Verification items for the finished model (mm, model axes). Face numbers are marked on the shaded views. A direction names the side the tool comes from. Give positions to 0.01 mm unless a question says otherwise; leave off trailing zeros. Write each loop counter-clockwise with the first axis right and the second up, starting at its lowest first coordinate (ties: lowest second). Pieces come first, ordered by that corner, then holes. Notation, with made-up numbers: (85.5, 87.25) - (99.5, 87.25) arc R28 cw to (99.5, 105.25) - close; hole circle Ø8 at (83.25, 79.25). An arc over 180 degrees is marked (long way). Answer as a JSON object with one key per item and string values. Group by question number.
Item 1: Sectioned sample at D-D, the plane x = -18. Record the boundary of the cut face in (y, z), and give its area (3 significant figures).
Item 2: Sectioned sample at B-B, the plane y = -31. Count the separate pieces of the cut face and the enclosed holes in it, and give its area (3 significant figures).
Item 3: Go/stop test with flat-tipped pins: pin 1 (3 mm diameter, centred on x = 11, z = -0.5, fed in from +Y); pin 2 (1.3 mm diameter, centred on y = -13.5, z = 0, fed in from -X); pin 3 (10 mm diameter, centred on x = -13.5, y = -12, fed in from -Z); pin 4 (2 mm diameter, centred on x = 6.5, y = -23, fed in from -Z). Record where each tip stops, or that it passes through.
Item 4: Tool access check on the marked faces 1 and 2. Record the directions out of +Z, -Z, +X, -X, +Y, -Y that give a thin tool (end or side, any length) a straight path to the whole face; none if there is none.
Item 5: Sectioned sample at C-C, the plane x = -9.5. Record the boundary of the cut face in (y, z).
Item 6: Sectioned sample at A-A, the plane z = -3.1. Record the boundary of the cut face in (x, y) (3 decimals), and give its area (3 significant figures).
Item 7: Scan lines: line 1 along Y through (x, z) = (9.5, 0.7); line 2 along Y through (x, z) = (22.5, -2.2); line 3 along Y through (x, z) = (-22, -3.05). Record each from-to range of solid material in increasing order. Write a range as [from, to].
```python
from build123d import *

# Parameters (mm, degrees)
F1_DEPTH    = 44.45
F2_R        = 5.07999
F3_R        = 1.397
F4_DEPTH    = 25.4
F5_W        = 15.24
F5_H        = 11.5777312835
F6_DEPTH    = 25.4
F7_R        = 2.54
F8_T1_DEPTH = 50.9820747894


# Not quite as in the source:
# - a fillet or chamfer that OpenCascade refuses, or shapes differently, is made with other operations: its cross-section is extruded or revolved along the edge and cut away or added
# - a fillet or chamfer is up to 0.001 mm smaller than in the source, because OpenCascade refuses the exact size


with BuildPart() as f1:
    # F0 (on Front) → F1 (new body)
    with BuildSketch(Plane.XZ):
        Polygon((0, 1.27), (-25.4, 1.27), (-25.4, -1.27), (-25.4, -3.81), (-19.05, -3.81), (-19.05, -1.27), (19.05, -1.27), (19.05, -3.81), (25.4, -3.81), (25.4, -1.27), (25.4, 1.27), align=None)
    extrude(amount=F1_DEPTH)

    # F2 (radius 5.08 in the source; OpenCascade refuses exactly that, so slightly less here)
    f2_edges = [f1.edges().sort_by_distance(p)[0] for p in [
        (-25.4, -22.225, 1.27),
        (25.4, -22.225, 1.27),
    ]]
    fillet(f2_edges, radius=F2_R)

    # F3 (on face) → F4 (cut)
    with BuildSketch(Plane(origin=(0, 0, -3.81), x_dir=(1, 0, 0), z_dir=(0, 0, -1))):
        with BuildLine():
            ThreePointArc((-22.225, 23.622), (-23.2128281733, 21.2371718267), (-20.828, 22.225))
            Line((-20.828, 22.225), (-22.225, 22.225))
            Line((-22.225, 22.225), (-22.225, 23.622))
        make_face()
        with BuildLine():
            Line((-22.225, 22.225), (-20.828, 22.225))
            ThreePointArc((-20.828, 22.225), (-21.2371718267, 23.2128281733), (-22.225, 23.622))
            Line((-22.225, 23.622), (-22.225, 22.225))
        make_face()
        with BuildLine():
            ThreePointArc((-22.225, 42.672), (-23.622, 41.275), (-22.225, 39.878))
            Line((-22.225, 39.878), (-22.225, 41.275))
            Line((-22.225, 41.275), (-22.225, 42.672))
        make_face()
        with BuildLine():
            Line((-22.225, 41.275), (-22.225, 39.878))
            ThreePointArc((-22.225, 39.878), (-21.2371718267, 40.2871718267), (-20.828, 41.275))
            ThreePointArc((-20.828, 41.275), (-21.2371718267, 42.2628281733), (-22.225, 42.672))
            Line((-22.225, 42.672), (-22.225, 41.275))
        make_face()
        with Locations((-22.225, 3.175)):
            Circle(F3_R)
        with Locations((22.225, 41.275)):
            Circle(F3_R)
        with Locations((22.225, 3.175)):
            Circle(F3_R)
        with Locations((22.225, 22.225)):
            Circle(F3_R)
    extrude(amount=-F4_DEPTH, mode=Mode.SUBTRACT)

    # F5 (on face) → F6 (cut)
    with BuildSketch(Plane.XY.offset(1.27)):
        with Locations((11.43, -12.1388656418)):
            Rectangle(F5_W, F5_H)
        with Locations((-11.43, -12.1388656418)):
            Rectangle(F5_W, F5_H)
        with Locations((11.43, -32.3111343582)):
            Rectangle(F5_W, F5_H)
        with Locations((-11.43, -32.3111343582)):
            Rectangle(F5_W, F5_H)
    extrude(amount=-F6_DEPTH, mode=Mode.SUBTRACT)

    # F7
    f7_edges = [f1.edges().sort_by_distance(p)[0] for p in [
        (-19.05, -6.35, 0),
        (-3.81, -17.927731, 0),
        (-3.81, -6.35, 0),
        (-19.05, -17.927731, 0),
        (-19.05, -38.1, 0),
        (3.81, -38.1, 0),
        (3.81, -17.927731, 0),
        (3.81, -6.35, 0),
        (-19.05, -26.522269, 0),
        (3.81, -26.522269, 0),
        (19.05, -26.522269, 0),
        (-3.81, -26.522269, 0),
        (19.05, -6.35, 0),
        (19.05, -17.927731, 0),
        (19.05, -38.1, 0),
        (-3.81, -38.1, 0),
    ]]
    fillet(f7_edges, radius=F7_R)

    # F8: chamfer of 1.27 on 14 edges, made by hand

    # F8_s2 → F8_t1 (cut)
    with BuildSketch(Plane.XZ.offset(-3.2660373947)):
        Polygon((19.05, -2.54), (20.32, -3.81), (19.05, -3.81), align=None)
        Polygon((-19.05, -2.54), (-20.32, -3.81), (-19.05, -3.81), align=None)
    extrude(amount=F8_T1_DEPTH, mode=Mode.SUBTRACT)


solid = f1.part
```
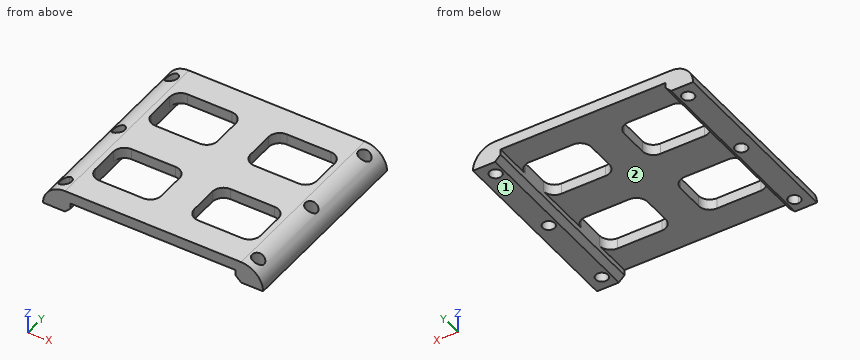
Geometry check:
{
 "1": {"outline": "(-44.45, -1.27) - (-37.62, -1.27) - (-37.62, 1.27) - (-44.45, 1.27) - close; (-27.01, -1.27) - (-17.44, -1.27) - (-17.44, 1.27) - (-27.01, 1.27) - close; (-6.83, -1.27) - (0, -1.27) - (0, 1.27) - (-6.83, 1.27) - close", "area": "59.0 mm^2"},
 "2": {"separate pieces": "3", "enclosed holes": "0", "area": "71.2 mm^2"},
 "3": {"pin 1": "y = 0", "pin 2": "x = -24.3", "pin 3": "through", "pin 4": "z = -1.27"},
 "4": {"face 1": "-Z, +X, -X, +Y, -Y", "face 2": "-Z, +Y, -Y"},
 "5": {"outline": "(-44.45, -1.27) - (-38.1, -1.27) - (-38.1, 1.27) - (-44.45, 1.27) - close; (-26.52, -1.27) - (-17.93, -1.27) - (-17.93, 1.27) - (-26.52, 1.27) - close; (-6.35, -1.27) - (0, -1.27) - (0, 1.27) - (-6.35, 1.27) - close"},
 "6": {"outline": "(-25.35, -44.45) - (-19.61, -44.45) - (-19.61, 0) - (-25.35, 0) - close; (19.61, -44.45) - (25.35, -44.45) - (25.35, 0) - (19.61, 0) - close; hole circle Ø2.794 at (-22.225, -41.275); hole circle Ø2.794 at (-22.225, -22.225); hole circle Ø2.794 at (-22.225, -3.175); hole circle Ø2.794 at (22.225, -41.275); hole circle Ø2.794 at (22.225, -22.225); hole circle Ø2.794 at (22.225, -3.175)", "area": "474 mm^2"},
 "7": {"line 1": "[-44.45, -38.1], [-26.52, -17.93], [-6.35, 0]", "line 2": "[-44.45, -42.64], [-39.91, -23.59], [-20.86, -4.54], [-1.81, 0]", "line 3": "[-44.45, -42.65], [-39.9, -23.6], [-20.85, -4.55], [-1.8, 0]"}
}
